from build123d import *

# Parameters (mm, degrees)
SKETCH_2_R          = 1
EXTRUDE_1_DEPTH     = 2.5
CUT_EXTRUDE_1_DEPTH = 10
FILLET_1_R          = 10


with BuildPart() as part:
    # 草图2 → 凸台-拉伸1 (new body)
    with BuildSketch(Plane(origin=(0, 0, 0), x_dir=(1, 0, 0), z_dir=(0, 1, 0))):
        with BuildLine():
            Line((14.476416474, 15.856761921), (14.874238191, 15.898449826))
            ThreePointArc((14.874238191, 15.898449826), (13.617518302, 17.223579787), (12.012278006, 16.352650461))
            Line((12.012278006, 16.352650461), (12.377645672, 16.189842387))
            ThreePointArc((12.377645672, 16.189842387), (12.736119234, 16.632239525), (13.267765014, 16.836129905))
            ThreePointArc((13.267765014, 16.836129905), (14.074924495, 16.596765827), (14.476416474, 15.856761921))
        make_face()
        with BuildLine():
            ThreePointArc((13.267765014, 16.836129905), (13.948344657, 16.54497389), (14.058411092, 15.812958962))
            Line((14.058411092, 15.812958962), (14.476416474, 15.856761921))
            ThreePointArc((14.476416474, 15.856761921), (14.074924495, 16.596765827), (13.267765014, 16.836129905))
        make_face()
        with BuildLine():
            Line((8.01763809, 14.922232709), (7.5, 12.990381057))
            Line((7.5, 12.990381057), (23.780514318, 10.680802356))
            ThreePointArc((23.780514318, 10.680802356), (26.918139154, 13.705908304), (23.893033206, 16.84353314))
            Line((23.893033206, 16.84353314), (14.874238191, 15.898449826))
            Line((14.874238191, 15.898449826), (14.476416474, 15.856761921))
            Line((14.476416474, 15.856761921), (14.058411092, 15.812958962))
            Line((14.058411092, 15.812958962), (5.923249556, 14.96047197))
            ThreePointArc((5.923249556, 14.96047197), (6.971617953, 15.005660189), (8.01763809, 14.922232709))
        make_face()
        with Locations((23.836773762, 13.762167748)):
            Circle(SKETCH_2_R, mode=Mode.SUBTRACT)
        with BuildLine():
            ThreePointArc((3.882285677, 14.488887394), (5.923249556, 14.96047197), (8.01763809, 14.922232709))
            Line((8.01763809, 14.922232709), (7.5, 12.990381057))
            ThreePointArc((7.5, 12.990381057), (5.405611466, 13.028620317), (3.364647586, 12.557035742))
            Line((3.364647586, 12.557035742), (3.882285677, 14.488887394))
        make_face()
    extrude(amount=EXTRUDE_1_DEPTH)

    # 草图3 → 切除-拉伸1 (cut)
    with BuildSketch(Plane(origin=(0, 2.5, 0), x_dir=(1, 0, 0), z_dir=(0, 1, 0))):
        Polygon((3.623466631, 13.522961568), (3.851948064, 12.718387546), (3.364647586, 12.557035742), align=None)
    extrude(amount=-CUT_EXTRUDE_1_DEPTH, mode=Mode.SUBTRACT)

    # 圆角1
    fillet_1_edges = [part.edges().sort_by_distance(p)[0] for p in [
        (14.874238191, 1.25, -15.898449826),
    ]]
    fillet(fillet_1_edges, radius=FILLET_1_R)


solid = part.part
Can you work these out from the model? Positions are in its coordinate system, mm. A direction names the side the tool comes from. Coordinates: 2 decimals unless noted, no trailing zeros. Loops run counter-clockwise (first coordinate to the right, second up) from the corner with the lowest first, then second, coordinate; pieces in that order, holes last. Notation, with made-up numbers: M -37.75,60.5 L 0.25,60.5 A20 cw 0.25,82.5 Z; hole C -14.75,83 d10. An arc over 180 degrees is marked long. Answer as CSV lines item,"result". Start each with the question number.
1. For faces 4 (the face through (10.048, 1.232, -15.393)), 5 (the face through (13.9, 1.2, -16.6)), 6 (the face through (18, 2.5, -14)), 7 (the face through (5.687, 1.232, -13.053)), 8 (the face through (21.496, 1.232, -16.592)), which set-ups out of +Z, -Z, +X, -X, +Y, -Y let a thin tool reach every point of the face, with its end or its side?
2. Suppose I cut it at C-C, the plane x = 19.25. List the corners of the cut face in (y, z) for me, plus the area to 3 significant figures.
3. For pin 1 Ø1.5 at (y, z) = (2, -15.5) entering from +X; pin 2 Ø1.8 at (x, z) = (23.84, -13.76) entering from +Y, each with a flat end and sliding along its axis, tell me the tip position at first contact or that it passes through.
4. Suppose I cut it at A-A, the plane z = -14.25. List the corners of the cut face in (x, y) for me, plus the area to 3 significant figures.
5. Suppose I cut it at B-B, the plane y = 1.1. List the corners of the cut face in (x, z) for me.
6. Suppose I cut it at D-D, the plane z = -11.5. List the corners of the cut face in (x, y) for me.
7. Thinking about a two-plate mould opening in Z: for faces 1 (the face through (4.874, 1.232, -14.784)), 2 (the face through (3.736, 1.268, -13.126)), 3 (the face through (12.73, 1.23, -16.63)), which applies, +Z half, -Z half, draft (parallel to the pull), parting line (faces both ways), or undercut?
8. If I drill on probe 1 along Z at (x, y) = (24, 0.8); probe 2 along X at (y, z) = (2.2, -13.5); probe 3 along X at (y, z) = (0.85, -13.25), over which ranges is the centre line in solid material (lowest first)? Write a range as [from, to].
Output:
1,face 4,"-X, +Y, -Y"
1,face 5,"+Y, -Y"
1,face 6,"+Z, -Z, +X, -X, +Y"
1,face 7,"+Z, +Y, -Y"
1,face 8,"-Z, +Y, -Y"
2,outline,"M 0,-16.36 L 2.5,-16.36 L 2.5,-11.32 L 0,-11.32 Z"
2,area,"12.6 mm^2"
3,pin 1,"stops at x = 26.76"
3,pin 2,"passes through"
4,outline,"M 3.82,0 L 22.96,0 L 22.96,2.5 L 3.82,2.5 Z; M 24.71,0 L 26.88,0 L 26.88,2.5 L 24.71,2.5 Z"
4,area,"53.3 mm^2"
5,outline,"M 3.62,-13.52 L 3.88,-14.49 A8.56 ccw 5.92,-14.96 L 14.06,-15.81 A0.76 cw 13.27,-16.84 A1.1 cw 12.38,-16.19 L 12.01,-16.35 A1.5 ccw 13.98,-17.12 A10 cw 19.03,-16.33 L 23.89,-16.84 A3.08 ccw 23.78,-10.68 L 7.5,-12.99 A8.56 cw 3.85,-12.72 Z; hole C 23.84,-13.76 d2"
6,outline,"M 18.01,0 L 25.93,0 L 25.93,2.5 L 18.01,2.5 Z"
7,face 1,"-Z half"
7,face 2,"+Z half"
7,face 3,"undercut"
8,probe 1,"z = [-16.84, -14.75], [-12.78, -10.68]"
8,probe 2,"x = [3.63, 22.87], [24.8, 26.91]"
8,probe 3,"x = [3.7, 22.98], [24.7, 26.88]"
